The model under review builds one solid part; all positions refer to its coordinate system, in mm. Face numbers are marked on the shaded views. A direction names the side the tool comes from. Round coordinates to 2 decimals unless told otherwise and drop trailing zeros. Write each loop counter-clockwise with the first axis right and the second up, starting at its lowest first coordinate (ties: lowest second). Pieces come first, ordered by that corner, then holes. Notation, with made-up numbers: (22.5, 56.5) - (44.5, 56.5) arc R10 ccw to (44.5, 60.5) - close; hole circle Ø9 at (59.25, 87.5). An arc over 180 degrees is marked (long way). Use one line per item in the form item = value.
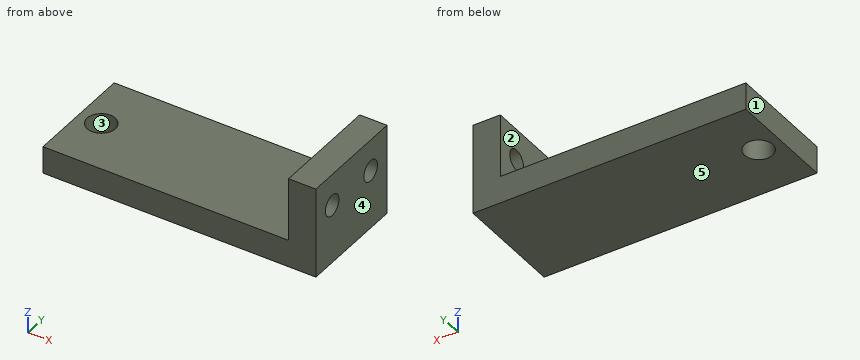
from build123d import *

# Parameters (mm, degrees)
F0_W     = 30
F0_H     = 12
F0_R     = 1.55
F1_DEPTH = 3
F2_W     = 12
F2_H     = 10
F2_R     = 1.15
F3_DEPTH = 3


with BuildPart() as f1:
    # F0 (on Top) → F1 (new body)
    with BuildSketch(Plane.XY):
        Rectangle(F0_W, F0_H)
        with Locations((-12.5, 0)):
            Circle(F0_R, mode=Mode.SUBTRACT)
    extrude(amount=F1_DEPTH)

    # F2 (on face) → F3 (join)
    with BuildSketch(Plane.YZ.offset(15)):
        with Locations((0, 5)):
            Rectangle(F2_W, F2_H)
        with Locations((-3.25, 6.5)):
            Circle(F2_R, mode=Mode.SUBTRACT)
        with Locations((3.25, 6.5)):
            Circle(F2_R, mode=Mode.SUBTRACT)
    extrude(amount=-F3_DEPTH)


solid = f1.part
(1) Add section D-D on y = -3.25. Write out the cut boundary in (x, z).
Geometry results:
outline = (-15, 0) - (15, 0) - (15, 5.35) - (12, 5.35) - (12, 3) - (-15, 3) - close; (12, 7.65) - (15, 7.65) - (15, 10) - (12, 10) - close
(2) The part is to be moulded in two halves that separate along X. For the marked faces 3, 4 and 5, say which applies: +X half, -X half, draft (parallel to the pull), parting line (faces both ways), or undercut.
Geometry results:
face_3 = undercut
face_4 = +X half
face_5 = draft
(3) Machinability: for the marked faces 1 and 2, which of the approach directions +Z, -Z, +X, -X, +Y, -Y give a long, thin tool a straight path to every point of the face, cutting with its end or side? Answer none if there is none.
Geometry results:
face_1 = +Z, -Z, -X, +Y, -Y
face_2 = +Z, -X, +Y, -Y
(4) Insertion check: P1, Ø6, axis at x = -7.5, y = 0, coming from the +Z side; P2, Ø2, axis at y = 2.5, z = 5, coming from the -X side. Each pin has a flat end and moves straight along its axis. Give the tip position at first contact, or say it passes through.
Geometry results:
P1 = 3
P2 = 12
(5) Add section A-A on z = 6.5. Write out the cut boundary in (x, y), then the cut area to 3 significant figures.
Geometry results:
outline = (12, -6) - (15, -6) - (15, -4.4) - (12, -4.4) - close; (12, -2.1) - (15, -2.1) - (15, 2.1) - (12, 2.1) - close; (12, 4.4) - (15, 4.4) - (15, 6) - (12, 6) - close
area = 22.2 mm2
(6) Add section B-B on y = 0. Write out the cut boundary in (x, z).
Geometry results:
outline = (-15, 0) - (-14.05, 0) - (-14.05, 3) - (-15, 3) - close; (-10.95, 0) - (15, 0) - (15, 10) - (12, 10) - (12, 3) - (-10.95, 3) - close
(7) To check wall thickness, follow L1, parallel to Z at x = 13, y = -3.25; L2, parallel to Y at x = -12.5, z = 1.45; L3, parallel to Z at x = -8.25, y = -0.5. State the ranges of each line that lie inside material, in increasing order.
Geometry results:
L1 = 0 to 5.35, 7.65 to 10
L2 = -6 to -1.55, 1.55 to 6
L3 = 0 to 3
(8) Add section C-C on x = -12.5. Write out the cut boundary in (y, z), then the cut area to 3 significant figures.
Geometry results:
outline = (-6, 0) - (-1.55, 0) - (-1.55, 3) - (-6, 3) - close; (1.55, 0) - (6, 0) - (6, 3) - (1.55, 3) - close
area = 26.7 mm2
